Study the drawing (mm; zero at the part's minimum x, y, z) and answer. A direction names the side the tool comes from. Round coordinates to 2 decimals unless told otherwise and drop trailing zeros. Write each loop counter-clockwise with the first axis right and the second up, starting at its lowest first coordinate (ties: lowest second). Pieces come first, ordered by that corner, then holes. Notation, with made-up numbers: (76, 23.25) -> (92, 23.25) arc R25 ccw to (92, 42.25) -> close; hole circle Ø1 at (15, 26). An arc over 180 degrees is marked (long way). Write each question's results on one line, items separated by ' | '. Start each with the question number.
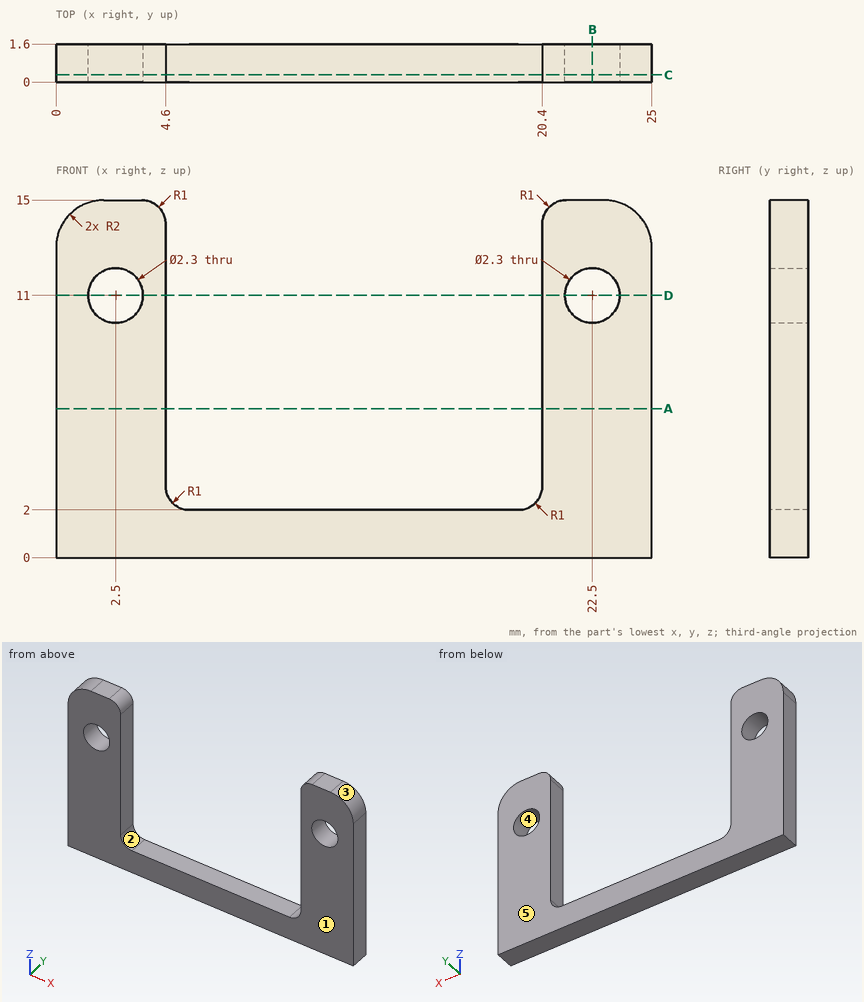
Q1. The part is cut by section C-C, the plane y = 0.3. Write down the section's boundary in (x, z), then the cut area to 3 significant figures.
Q2. Determine the mould class of the marked faces 3, 4 and 5 for opening direction X: pulls with the +X half, pulls with the -X half, needs draft (parallel to the pull), parting line crosses it, or undercut.
Q3. The part is cut by section B-B, the plane x = 22.5. Write down the section's boundary in (y, z).
Q4. For the marked faces 1 and 2, determine the directions among +Z, -Z, +X, -X, +Y, -Y from which every point of the face is accessible in a straight line to the end or side of a thin tool.
Q5. The part is cut by section D-D, the plane z = 11. Write down the section's boundary in (x, y), then the cut area to 3 significant figures.
Q6. The part is cut by section A-A, the plane z = 6.25. Write down the section's boundary in (x, y).
Q7. Find the intervals of material crossed by line 1 (X direction, y = 0.45, z = 11); line 2 (X direction, y = 0.8, z = 4.5); line 3 (Z direction, x = 2.5, y = 1), in increasing order.
Q8. This flat-tipped pin is pushed along its axis until it touches: pin 1 (3.5 mm diameter, centred on x = 2.5, z = 11, fed in from -Y). Where does it stop, or does it pass through?
Answers follow:
1) outline: (0, 0) -> (25, 0) -> (25, 13) arc R2 ccw to (23, 15) -> (21.4, 15) arc R1 ccw to (20.4, 14) -> (20.4, 3) arc R1 cw to (19.4, 2) -> (5.6, 2) arc R1 cw to (4.6, 3) -> (4.6, 14) arc R1 ccw to (3.6, 15) -> (2, 15) arc R2 ccw to (0, 13) -> close; hole circle Ø2.3 at (2.5, 11); hole circle Ø2.3 at (22.5, 11) | area: 160 mm^2
2) face 3: pulls with the +X half | face 4: undercut | face 5: needs draft
3) outline: (0, 0) -> (1.6, 0) -> (1.6, 9.85) -> (0, 9.85) -> close; (0, 12.15) -> (1.6, 12.15) -> (1.6, 15) -> (0, 15) -> close
4) face 1: +Z, -Z, +X, -X, -Y | face 2: +Z, +Y, -Y
5) outline: (0, 0) -> (1.35, 0) -> (1.35, 1.6) -> (0, 1.6) -> close; (3.65, 0) -> (4.6, 0) -> (4.6, 1.6) -> (3.65, 1.6) -> close; (20.4, 0) -> (21.35, 0) -> (21.35, 1.6) -> (20.4, 1.6) -> close; (23.65, 0) -> (25, 0) -> (25, 1.6) -> (23.65, 1.6) -> close | area: 7.36 mm^2
6) outline: (0, 0) -> (4.6, 0) -> (4.6, 1.6) -> (0, 1.6) -> close; (20.4, 0) -> (25, 0) -> (25, 1.6) -> (20.4, 1.6) -> close
7) line 1: 0 to 1.35, 3.65 to 4.6, 20.4 to 21.35, 23.65 to 25 | line 2: 0 to 4.6, 20.4 to 25 | line 3: 0 to 9.85, 12.15 to 15
8) pin 1: y = 0
